Check sheet for the drawn part. Datum: minimum x, y, z corner. Units: mm. A direction names the side the tool comes from. Coordinates: 2 decimals unless noted, no trailing zeros. Loops run counter-clockwise (first coordinate to the right, second up) from the corner with the lowest first, then second, coordinate; pieces in that order, holes last. Notation, with made-up numbers: M 39,45.25 L 84,45.25 A18 ccw 84,66.25 Z; hole C -10,-13 d5. An arc over 180 degrees is marked long. Use CSV: the item, a comma, the result in double quotes. Start each with the question number.
(1) Set-up check for the marked faces 5 and 6: record each of +Z, -Z, +X, -X, +Y, -Y from which the full face is reachable in a straight line by a thin tool's end or side.
(2) Section check C-C on z = 11. Record the cut outline in (x, y).
(3) Scan lines: line 1 (Z direction, x = 22.75, y = 7.5); line 2 (X direction, y = 12.25, z = 1.25); line 3 (Y direction, x = 25.5, z = 11). Record each from-to range of solid material in increasing order.
(4) Section check D-D on x = 23.5. Record the cut outline in (y, z).
(5) Section check A-A on y = 16.5. Record the cut outline in (x, z).
(6) Section check B-B on x = 5. Record the cut outline in (y, z).
(7) Go/stop test with flat-tipped pins: pin 1 Ø4 at (y, z) = (16.5, 11) entering from -X; pin 2 Ø5 at (x, y) = (18.5, 7.5) entering from +Z; pin 3 Ø4 at (x, z) = (5, 3.5) entering from +Y; pin 4 Ø3 at (x, z) = (23, 10) entering from -Y. Record where each tip stops, or that it passes through.
(8) Draft check along Z on the marked faces 1, 2, 3 and 4. Enter one of: pulls with the +Z half, pulls with the -Z half, needs draft (parallel to the pull), parting line crosses it, or undercut.
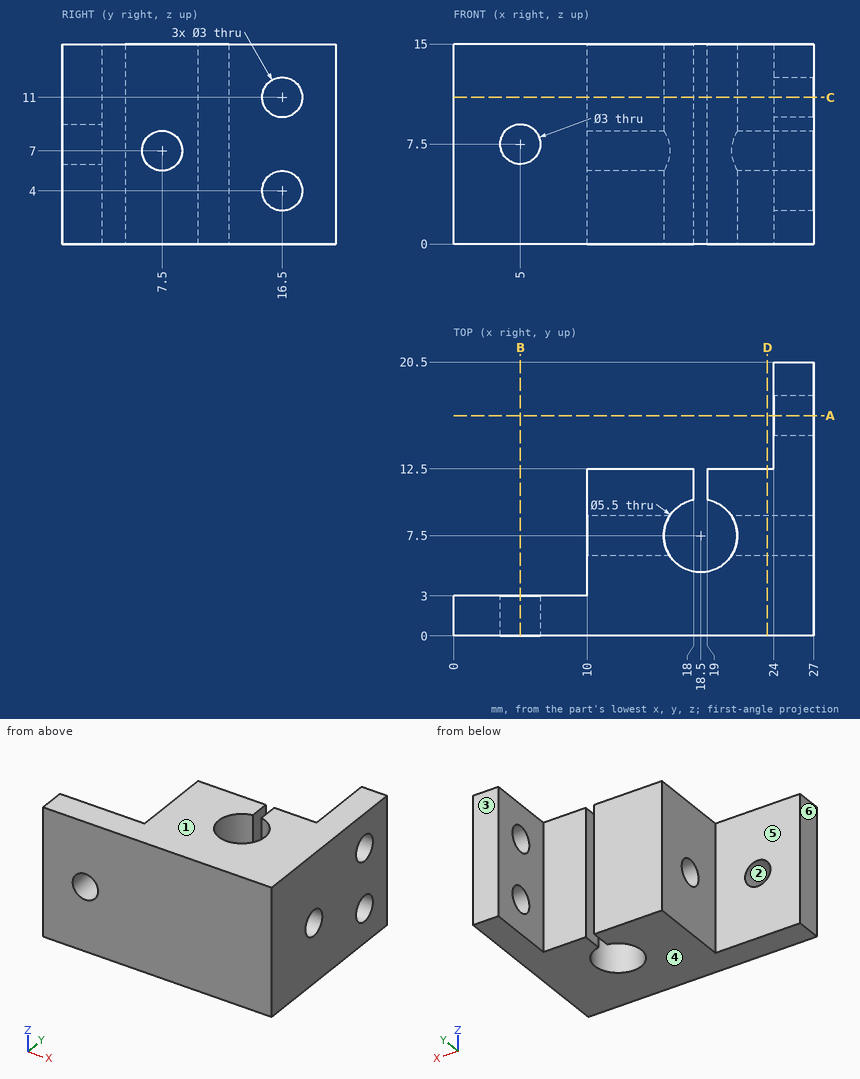
Outcome:
1,face 5,"+Z, -Z, -X, +Y"
1,face 6,"+Z, -Z, -X, +Y, -Y"
2,outline,"M 0,0 L 27,0 L 27,15 L 24,15 L 24,12.5 L 19,12.5 L 19,10.2 A2.75 cw long 18,10.2 L 18,12.5 L 10,12.5 L 10,3 L 0,3 Z; M 24,18 L 27,18 L 27,20.5 L 24,20.5 Z"
3,line 1,"z = 0 to 5.5, 8.5 to 15"
3,line 2,"x = 10 to 18, 19 to 27"
3,line 3,"y = 0 to 15, 18 to 20.5"
4,outline,"M 0,0 L 12.5,0 L 12.5,15 L 0,15 Z; hole C 7.5,7 d3"
5,outline,"M 24,0 L 27,0 L 27,2.5 L 24,2.5 Z; M 24,5.5 L 27,5.5 L 27,9.5 L 24,9.5 Z; M 24,12.5 L 27,12.5 L 27,15 L 24,15 Z"
6,outline,"M 0,0 L 3,0 L 3,6 L 0,6 Z; M 0,9 L 3,9 L 3,15 L 0,15 Z"
7,pin 1,"stops at x = 24"
7,pin 2,"passes through"
7,pin 3,"stops at y = 3"
7,pin 4,"stops at y = 0"
8,face 1,"pulls with the +Z half"
8,face 2,"undercut"
8,face 3,"needs draft"
8,face 4,"pulls with the -Z half"
